Design review of the part built by this model. Coordinates are the model's own, in mm. Give positions to 0.01 mm unless a question says otherwise; leave off trailing zeros. Write each loop counter-clockwise with the first axis right and the second up, starting at its lowest first coordinate (ties: lowest second). Pieces come first, ordered by that corner, then holes. Notation, with made-up numbers: (85.25, 84.5) -> (89.25, 84.5) arc R21 ccw to (89.25, 108.5) -> close; hole circle Ø11 at (-20, 0). An arc over 180 degrees is marked (long way). Return JSON: item names as keys, results as strings. Group by question number.
Autodesk Inventor part; units mm, degrees
ref_plane "YZ Plane" through (0, 0, 0) normal (1, 0, 0) x (0, 1, 0)
ref_plane "XZ Plane" through (0, 0, 0) normal (0, 1, 0) x (-1, 0, 0)
ref_plane "XY Plane" through (0, 0, 0) normal (0, 0, 1) x (1, 0, 0)
sketch "Szkic1" plane through (0, 0, 0) normal (0, 1, 0) x (-1, 0, 0)
  line L0 (38.1, 143.51) -> (30.48, 143.51)
  line L1 (27.94, 140.97) -> (27.94, 2.54)
  line L2 (25.4, 0) -> (2.54, 0)
  line L3 (0, 2.54) -> (0, 140.97)
  line L4 (-2.54, 143.51) -> (-10.16, 143.51)
  line L5 (-12.7, 140.97) -> (-12.7, -63.5)
  line L6 (-10.16, -66.04) -> (-2.54, -66.04)
  line L7 (0, -63.5) -> (0, -15.24)
  line L8 (2.54, -12.7) -> (38.1, -12.7)
  line L9 (40.64, -10.16) -> (40.64, 140.97)
  line L10 (34.29, 143.51) -> (34.29, -12.7) construction
  line L11 (-6.35, -66.04) -> (-6.35, 143.51) construction
  circle A0 centre (34.29, -6.35) radius 1.6
  circle A1 centre (-6.35, -6.35) radius 1.6
  circle A2 centre (34.29, 29.21) radius 1.6
  circle A3 centre (-6.35, 29.21) radius 1.6
  circle A4 centre (34.29, 64.77) radius 1.6
  circle A5 centre (-6.35, 64.77) radius 1.6
  circle A6 centre (34.29, 100.33) radius 1.6
  circle A7 centre (-6.35, 100.33) radius 1.6
  circle A8 centre (34.29, 135.89) radius 1.6
  circle A9 centre (-6.35, 135.89) radius 1.6
  circle A10 centre (-6.35, -58.42) radius 1.6
  line L12 (40.64, -10.16) -> (38.1, -12.7)
  line L13 (25.4, 0) -> (27.94, 2.54)
  line L14 (2.54, -12.7) -> (0, -15.24)
  line L15 (0, 2.54) -> (2.54, 0)
  line L16 (-2.54, -66.04) -> (0, -63.5)
  line L17 (-10.16, -66.04) -> (-12.7, -63.5)
  line L18 (-2.54, 143.51) -> (0, 140.97)
  line L19 (-10.16, 143.51) -> (-12.7, 140.97)
  line L20 (27.94, 140.97) -> (30.48, 143.51)
  line L21 (38.1, 143.51) -> (40.64, 140.97)
  line L22 (19.05, 0) -> (19.05, -6.35) construction
  line L23 (19.05, -6.35) -> (19.05, -12.7) construction
  line L24 (19.05, -6.35) -> (34.29, -6.35) construction
  line L25 (19.05, -6.35) -> (-6.35, -6.35) construction
  line L26 (39.64, 140.5558) -> (37.6858, 142.51)
  line L27 (37.6858, 142.51) -> (30.8942, 142.51)
  line L28 (30.8942, 142.51) -> (28.94, 140.5558)
  line L29 (28.94, 140.5558) -> (28.94, 2.1258)
  line L30 (28.94, 2.1258) -> (25.8142, -1)
  line L31 (25.8142, -1) -> (2.1258, -1)
  line L32 (2.1258, -1) -> (-1, 2.1258)
  line L33 (-1, 2.1258) -> (-1, 140.5558)
  line L34 (-1, 140.5558) -> (-2.9542, 142.51)
  line L35 (-2.9542, 142.51) -> (-9.7458, 142.51)
  line L36 (-9.7458, 142.51) -> (-11.7, 140.5558)
  line L37 (-11.7, 140.5558) -> (-11.7, -63.0858)
  line L38 (-11.7, -63.0858) -> (-9.7458, -65.04)
  line L39 (-9.7458, -65.04) -> (-2.9542, -65.04)
  line L40 (-2.9542, -65.04) -> (-1, -63.0858)
  line L41 (-1, -63.0858) -> (-1, -14.8258)
  line L42 (-1, -14.8258) -> (2.1258, -11.7)
  line L43 (2.1258, -11.7) -> (37.6858, -11.7)
  line L44 (37.6858, -11.7) -> (39.64, -9.7458)
  line L45 (39.64, -9.7458) -> (39.64, 140.5558)
  point P0 (0, 0)
  point P1 (40.64, 143.51)
  point P2 (27.94, 143.51)
  point P3 (27.94, 0)
  point P4 (0, 0)
  point P5 (0, 143.51)
  point P6 (-12.7, 143.51)
  point P7 (-12.7, -66.04)
  point P8 (0, -66.04)
  point P9 (0, -12.7)
  point P10 (40.64, -12.7)
  dimension "d0" = 12.7
  dimension "d1" = 209.55
  dimension "d2" = 156.21
  dimension "d3" = 27.94
  dimension "d4" = 3.2
  dimension "d5" = 3.2
  dimension "d8" = 35.56
  dimension "d13" = 3.2
  dimension "d14" = 7.62
  dimension "d16" = 2.54
  dimension "d17" = 2.54
  dimension "d18" = 2.54
  dimension "d19" = 2.54
  dimension "d20" = 2.54
  dimension "d21" = 2.54
  dimension "d22" = 2.54
  dimension "d23" = 2.54
  dimension "d24" = 2.54
  dimension "d25" = 2.54
  dimension "d26" = 2.54
  dimension "d27" = 2.54
  dimension "d28" = 2.54
  dimension "d29" = 2.54
  dimension "d30" = 2.54
  dimension "d31" = 2.54
  dimension "d32" = 2.54
  dimension "d33" = 2.54
  dimension "d34" = 2.54
  dimension "d35" = 2.54
  dimension "d36" = 12.7
  dimension "d37" = 1
sketch "Szkic2" plane through (0, 0, 0) normal (0, 1, 0) x (-1, 0, 0)
  point P0 (0, 0)
extrude "Wyciągnięcie proste1" add sketch "Szkic1" along normal blind 3 contours L45 L44 L43 L42 L41 L40 L39 L38 L37 L36 L35 L34 L33 L32 L31 L30 L29 L28 L27 L26
properties part number "bar_-BattPow"
Q1. Take a section at A-A, the plane z = 95. Give the boundary of the cut face in (x, y), plus the area to 3 significant figures.
Q2. Take a section at D-D, the plane z = -47.5. Give the boundary of the cut face in (x, y), plus the area to 3 significant figures.
Q3. Take a section at C-C, the plane x = -17.5. Give the boundary of the cut face in (y, z).
Q4. Take a section at B-B, the plane y = 2.35. Count the separate pieces of the cut face and the enclosed holes in it, plus the area to 3 significant figures.
Q5. For L1, parallel to Z at x = -34.29, y = 1.95; L2, parallel to X at y = 1.8, z = 135.89; L3, parallel to X at y = 2.4, z = 113, list the stretches that pass through material, from the lowest coordinate up. Write a range as from..to.
Final values:
{
 "1": {"outline": "(-39.64, 0) -> (-28.94, 0) -> (-28.94, 3) -> (-39.64, 3) -> close; (1, 0) -> (11.7, 0) -> (11.7, 3) -> (1, 3) -> close", "area": "64.2 mm²"},
 "2": {"outline": "(1, 0) -> (11.7, 0) -> (11.7, 3) -> (1, 3) -> close", "area": "32.1 mm²"},
 "3": {"outline": "(0, -11.7) -> (3, -11.7) -> (3, -1) -> (0, -1) -> close"},
 "4": {"separate pieces": "1", "enclosed holes": "11", "area": "4,100 mm²"},
 "5": {"L1": "z = -11.7..-7.95, -4.75..27.61, 30.81..63.17, 66.37..98.73, 101.93..134.29, 137.49..142.51", "L2": "x = -39.64..-35.89, -32.69..-28.94, 1..4.75, 7.95..11.7", "L3": "x = -39.64..-28.94, 1..11.7"}
}
